For this review, use the dimensioned drawing (mm, ordinates from the lowest corner) and the shaded views. A direction names the side the tool comes from. Coordinates: 2 decimals unless noted, no trailing zeros. Order: outer loops, then holes, each group sorted by start corner. A loop starts at its lowest first (then second) coordinate and runs counter-clockwise, first axis right, second up. Notation, with made-up numbers: M 56.25,84 L 74.25,84 A8 cw 74.25,92 Z; hole C -8.5,56.25 d2. An arc over 180 degrees is marked long. Answer in a Markdown table with one row per item.
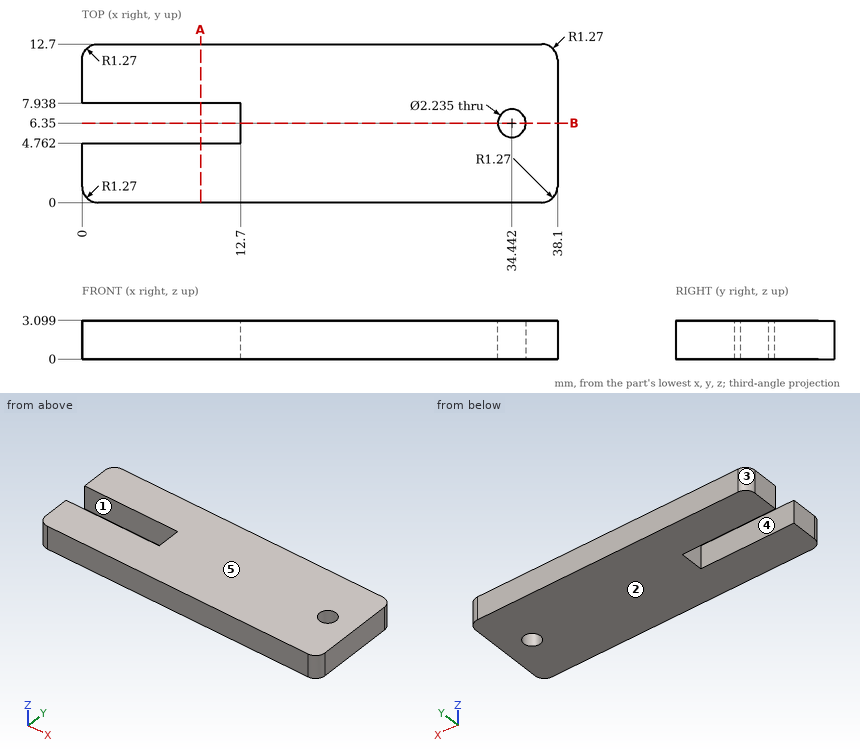
(1) Take a section at B-B (y = 6.35). Write out the cut boundary in (x, z) (1 decimal).
Report:
| item | result |
|---|---|
| outline | M 12.7,0 L 33.3,0 L 33.3,3.1 L 12.7,3.1 Z; M 35.6,0 L 38.1,0 L 38.1,3.1 L 35.6,3.1 Z |
(2) Insertion check: P1, Ø3.5, axis at x = 34.44, y = 6.35, coming from the +Z side; P2, Ø0.9, axis at y = 6.5, z = 1, coming from the -X side. Each pin has a flat end and moves straight along its axis. Give the tip position at first contact, or say it passes through.
Report:
| item | result |
|---|---|
| P1 | z = 3.1 |
| P2 | x = 12.7 |
(3) The part is to be moulded in two halves that separate along Y. For the marked faces 1, 2 and 3, say which applies: +Y half, -Y half, draft (parallel to the pull), parting line (faces both ways), or undercut.
Report:
| item | result |
|---|---|
| face 1 | undercut |
| face 2 | draft |
| face 3 | +Y half |
(4) Take a section at A-A (x = 9.5). Write out the cut boundary in (y, z), then the cut area to 3 significant figures.
Report:
| item | result |
|---|---|
| outline | M 0,0 L 4.76,0 L 4.76,3.1 L 0,3.1 Z; M 7.94,0 L 12.7,0 L 12.7,3.1 L 7.94,3.1 Z |
| area | 29.5 mm^2 |
(5) To check wall thickness, follow line 1 (Y direction, x = 11.5, z = 1.9); line 2 (Y direction, x = 34.5, z = 2.6) (1 decimal); line 3 (X direction, y = 6.75, z = 1.2) (1 decimal). State the ranges of each line that lie inside material, in increasing order. Write a range as [from, to].
Report:
| item | result |
|---|---|
| line 1 | [0, 4.76], [7.94, 12.7] |
| line 2 | [0, 5.2], [7.5, 12.7] |
| line 3 | [12.7, 33.4], [35.5, 38.1] |
(6) Machinability: for the marked faces 4 and 5, which of the approach directions +Z, -Z, +X, -X, +Y, -Y give a long, thin tool a straight path to every point of the face, cutting with its end or side? Answer none if there is none.
Report:
| item | result |
|---|---|
| face 4 | +Z, -Z, -X |
| face 5 | +Z, +X, -X, +Y, -Y |
